Solid Edge part; units mm, degrees
sketch "Sketch1" plane through (0, 0, 0) normal (0, 0, 1) x (1, 0, 0)
  line L0 (2.0207, 3.5) -> (-2.0207, 3.5)
  line L1 (-2.0207, 3.5) -> (-4.0415, 0)
  line L2 (-4.0415, 0) -> (-2.0207, -3.5)
  line L3 (-2.0207, -3.5) -> (2.0207, -3.5)
  line L4 (2.0207, -3.5) -> (4.0415, 0)
  line L5 (4.0415, 0) -> (2.0207, 3.5)
extrude "Protrusion1" add sketch "Sketch1" against normal blind 2.5
sketch "Sketch2" plane through (19.7841, 16.7997, -2.5) normal (0, 0, -1) x (1, 0, 0)
  circle A0 centre (-19.7841, 16.7997) radius 5
extrude "ExtrudedProtrusion_2" add sketch "Sketch2" against normal blind 0.5
sketch "Sketch3" plane through (19.7841, 16.7997, -2.5) normal (0, 0, -1) x (1, 0, 0)
  circle A0 centre (-19.7841, 16.7997) radius 2.5
extrude "ExtrudedProtrusion_3" add sketch "Sketch3" along normal blind 10
sketch "Sketch4" plane through (0, 0, 0) normal (0, -1, 0) x (1, 0, 0)
  line L0 (3.5, 0) -> (4.0415, 0)
  line L1 (4.0415, 0) -> (4.0415, -0.3126)
  line L2 (4.0415, -0.3126) -> (3.5, 0)
revolve "RevolvedCutout1" cut sketch "Sketch4" angle 360 about axis through (0, 0, 54) along (0, 0, -1)
Design review of the part built by this model. Coordinates are the model's own, in mm. A direction names the side the tool comes from. Give positions to 0.01 mm unless a question says otherwise; leave off trailing zeros. Write each loop counter-clockwise with the first axis right and the second up, starting at its lowest first coordinate (ties: lowest second). Pieces come first, ordered by that corner, then holes. Notation, with made-up numbers: M 19,75.25 L 72,75.25 A17 ccw 72,85.25 Z; hole C 56,75 d8. An arc over 180 degrees is marked long. Answer as a JSON object with one key per item and string values. Group by question number.
1) We need section A-A (y = -4). Give the boundary of the cut face in (x, z).
2) We need section B-B (z = -3.25). Give the boundary of the cut face in (x, y), and give its area (3 significant figures).
3) Tool access review of faces 1 (the face through (-3.045, -1.726, -0.986)), 2 (the face through (3.045, 1.726, -0.986)), 3 (the face through (3, -1.8, -1)), 4 (the face through (0, 3.5, -1)), 5 (the face through (0, -4, -2)): name each direction out of +Z, -Z, +X, -X, +Y, -Y from which nothing blocks a thin tool from reaching the whole face with its end or side.
4) For line 1 along Z through (x, y) = (-4.25, 1.5); line 2 along Z through (x, y) = (-1, 3.25); line 3 along Y through (x, z) = (2.75, -1), list the stretches that pass through material, from the lowest coordinate up.
5) Clearance check with flat-ended pins moving along their axes: pin 1 Ø1 at (x, z) = (0.5, -1) entering from -Y; pin 2 Ø2 at (x, z) = (0, -10) entering from -Y; pin 3 Ø2 at (y, z) = (-3.5, -2.5) entering from -X. State where each tip first meets the part, or that it passes through.
Answer key:
{
 "1": {"outline": "M -3,-2.5 L 3,-2.5 L 3,-2 L -3,-2 Z"},
 "2": {"outline": "C 0,0 d5", "area": "19.6 mm²"},
 "3": {"face 1": "+Z, -X, -Y", "face 2": "+Z, +X, +Y", "face 3": "+Z, +X, -Y", "face 4": "+Z, +X, -X, +Y", "face 5": "+Z"},
 "4": {"line 1": "z = -2.5 to -2", "line 2": "z = -2.5 to 0", "line 3": "y = -2.24 to 2.24"},
 "5": {"pin 1": "stops at y = -3.5", "pin 2": "stops at y = -2.5", "pin 3": "stops at x = -4.33"}
}
